Can you work these out from the drawing? Everything is in mm from the part's minimum corner. A direction names the side the tool comes from. Round coordinates to 2 decimals unless told otherwise and drop trailing zeros. Write each loop counter-clockwise with the first axis right and the second up, starting at its lowest first coordinate (ties: lowest second). Pieces come first, ordered by that corner, then holes. Notation, with made-up numbers: (76, 1) -> (96, 1) arc R19 ccw to (96, 32) -> close; hole circle Ø9 at (52, 85.25). An arc over 180 degrees is marked (long way). Answer as CSV lines item,"result".
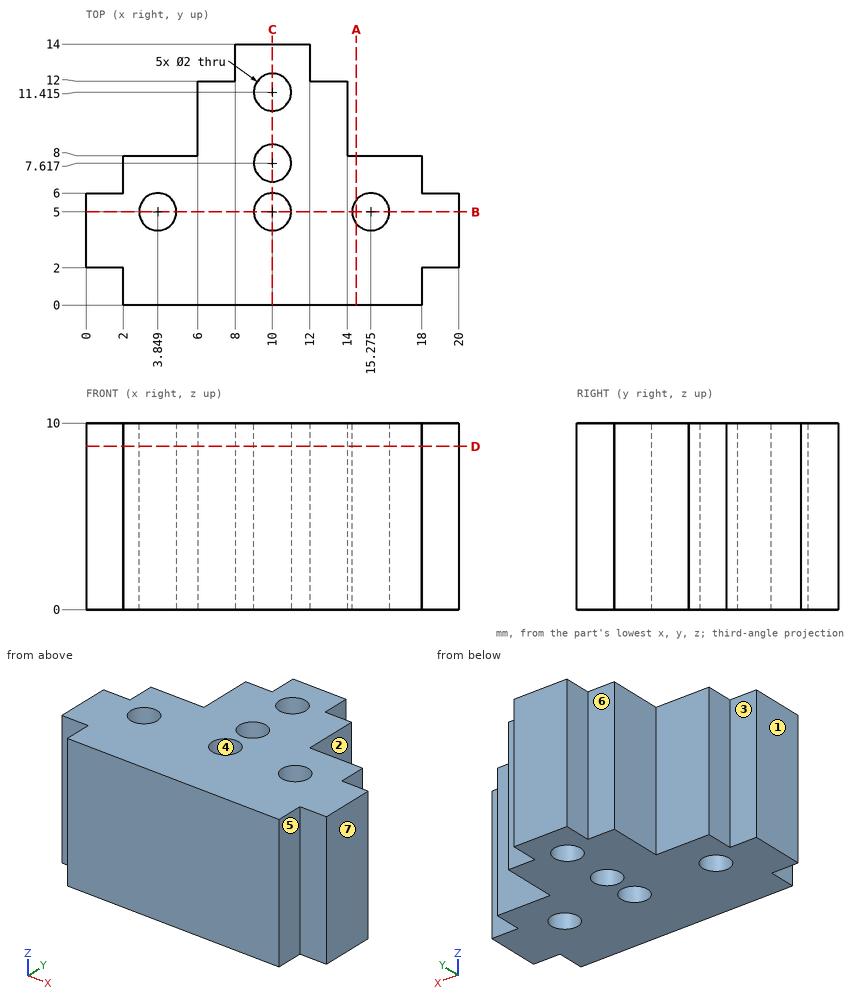
Item 1: Will these pins go through, and if not, where does the flat tip stop? pin 1 (2 mm diameter, centred on x = 4, z = 4.5, fed in from +Y); pin 2 (0.6 mm diameter, centred on y = 7.5, z = 7, fed in from +X); pin 3 (1.6 mm diameter, centred on x = 0.5, z = 3, fed in from +Y).
Results found:
pin 1,"stops at y = 8"
pin 2,"stops at x = 18"
pin 3,"stops at y = 6"
Item 2: For the marked faces 5, 6 and 7, which set-ups out of +Z, -Z, +X, -X, +Y, -Y let a thin tool reach every point of the face, with its end or its side?
Results found:
face 5,"+Z, -Z, +X, -Y"
face 6,"+Z, -Z, -X, +Y"
face 7,"+Z, -Z, +X, +Y, -Y"
Item 3: I need wall thicknesses on L1, parallel to Y at x = 10, z = 3 (1 decimal); L2, parallel to X at y = 4.5, z = 9.75 (1 decimal); L3, parallel to X at y = 9.75, z = 1.5. Which ranges of each line are inside material? Lowest first, please.
Results found:
L1,"y = 0 to 4, 6 to 6.6, 8.6 to 10.4, 12.4 to 14"
L2,"x = 0 to 3, 4.7 to 9.1, 10.9 to 14.4, 16.1 to 20"
L3,"x = 6 to 14"
Item 4: If we mould it in two halves opening along X, with no side actions, what happens to the marked faces 1, 2, 3 and 4? For each: pulls with the +X half, pulls with the -X half, needs draft (parallel to the pull), parting line crosses it, or undercut.
Results found:
face 1,"pulls with the -X half"
face 2,"pulls with the +X half"
face 3,"needs draft"
face 4,"undercut"
Item 5: Suppose I cut it at A-A, the plane x = 14.5. List the corners of the cut face in (y, z) for me.
Results found:
outline,"(0, 0) -> (4.37, 0) -> (4.37, 10) -> (0, 10) -> close; (5.63, 0) -> (8, 0) -> (8, 10) -> (5.63, 10) -> close"
Item 6: Suppose I cut it at D-D, the plane z = 8.75. List the corners of the cut face in (x, y) for me (1 decimal).
Results found:
outline,"(0, 2) -> (2, 2) -> (2, 0) -> (18, 0) -> (18, 2) -> (20, 2) -> (20, 6) -> (18, 6) -> (18, 8) -> (14, 8) -> (14, 12) -> (12, 12) -> (12, 14) -> (8, 14) -> (8, 12) -> (6, 12) -> (6, 8) -> (2, 8) -> (2, 6) -> (0, 6) -> close; hole circle Ø2 at (3.8, 5); hole circle Ø2 at (10, 5); hole circle Ø2 at (10, 7.6); hole circle Ø2 at (10, 11.4); hole circle Ø2 at (15.3, 5)"
Item 7: Suppose I cut it at B-B, the plane y = 5. List the corners of the cut face in (x, z) for me (1 decimal), then the cut area to 3 significant figures.
Results found:
outline,"(0, 0) -> (2.8, 0) -> (2.8, 10) -> (0, 10) -> close; (4.8, 0) -> (9, 0) -> (9, 10) -> (4.8, 10) -> close; (11, 0) -> (14.3, 0) -> (14.3, 10) -> (11, 10) -> close; (16.3, 0) -> (20, 0) -> (20, 10) -> (16.3, 10) -> close"
area,"140 mm²"
Item 8: Suppose I cut it at C-C, the plane x = 10. List the corners of the cut face in (y, z) for me (1 decimal).
Results found:
outline,"(0, 0) -> (4, 0) -> (4, 10) -> (0, 10) -> close; (6, 0) -> (6.6, 0) -> (6.6, 10) -> (6, 10) -> close; (8.6, 0) -> (10.4, 0) -> (10.4, 10) -> (8.6, 10) -> close; (12.4, 0) -> (14, 0) -> (14, 10) -> (12.4, 10) -> close"
